Here's how the part is built. I have some questions about the finished solid (model axes, mm). Coordinates: 2 decimals unless noted, no trailing zeros. Write each loop counter-clockwise with the first axis right and the second up, starting at its lowest first coordinate (ties: lowest second). Pieces come first, ordered by that corner, then holes.
Item 1: Please list where these lines run through material, in increasing order: line 1 (Z direction, x = -30, y = 2.25); line 2 (Z direction, x = -8, y = 1.1); line 3 (X direction, y = 1.9, z = 8).
Item 2: I'm going to push a flat-ended pin straight in: P1, Ø5, axis at x = -62, z = 11, coming from the +Y side. Where does the tip first touch, or does it pass through?
Item 3: I want a section at A-A (x = -8). Please give me the cut outline in (y, z), and give its area (3 significant figures).
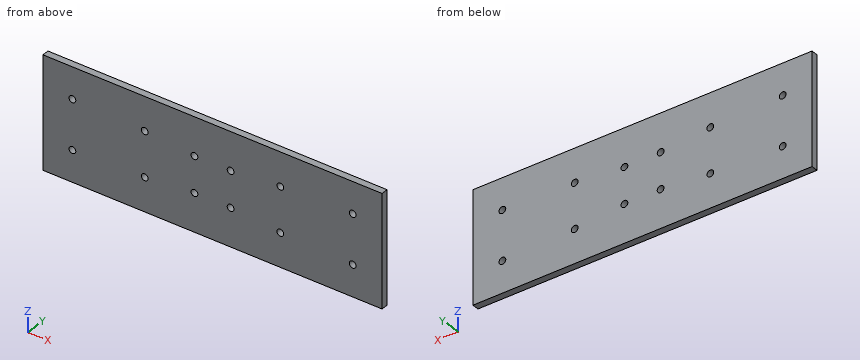
Autodesk Inventor part; units mm, degrees
ref_plane "YZ Plane" through (0, 0, 0) normal (1, 0, 0) x (0, 1, 0)
ref_plane "XZ Plane" through (0, 0, 0) normal (0, 1, 0) x (-1, 0, 0)
ref_plane "XY Plane" through (0, 0, 0) normal (0, 0, 1) x (1, 0, 0)
sketch "Szkic1" plane through (0, 0, 0) normal (0, 1, 0) x (-1, 0, 0)
  line L0 (75, 25) -> (-75, 25)
  line L1 (-75, 25) -> (-75, -25)
  line L2 (-75, -25) -> (75, -25)
  line L3 (75, -25) -> (75, 25)
  line L4 (75, 25) -> (-75, -25) construction
  line L5 (-75, 25) -> (75, -25) construction
  point P0 (0, 0)
  dimension "d0" = 150
  dimension "d1" = 50
extrude "Wyciągnięcie proste1" add sketch "Szkic1" along normal blind 3
sketch "Szkic3" plane through (0, 3, 0) normal (0, 1, 0) x (1, 0, 0)
  line L0 (75, 25) -> (-75, 25)
  line L1 (0, 25) -> (0, -25) construction
  line L2 (-75, -25) -> (75, -25)
  line L3 (-75, 25) -> (-75, -25)
  line L4 (-75, 0) -> (75, 0) construction
  line L5 (75, -25) -> (75, 25)
  point P0 (0, 0)
  point P1 (-30, 10)
  point P2 (30, 10)
  point P3 (-30, -10)
  point P4 (30, -10)
  dimension "d16" = 15
  dimension "d43" = 60
hole "Otwór2" at (-30, 3, -10) at (30, 3, -10) at (-30, 3, 10) at (30, 3, 10) direction (0, -1, 0) diameter 3 depth 8 tip angle 118
sketch "Szkic4" plane through (0, 3, 0) normal (0, 1, 0) x (1, 0, 0)
  line L0 (75, -25) -> (75, 25)
  line L1 (-75, 25) -> (-75, -25)
  line L2 (-75, 0) -> (75, 0) construction
  line L3 (75, 25) -> (-75, 25)
  line L4 (0, 25) -> (0, -25) construction
  point P0 (0, 0)
  point P1 (62, 11)
  point P2 (62, -11)
  point P3 (-62, 11)
  point P4 (-62, -11)
  dimension "d24" = 13
  dimension "d25" = 11
hole "Otwór3" at (62, 3, -11) at (62, 3, 11) at (-62, 3, -11) at (-62, 3, 11) direction (0, -1, 0) diameter 3 depth 8 tip angle 118
sketch "Szkic5" plane through (0, 3, 0) normal (0, 1, 0) x (1, 0, 0)
  line L0 (-8, -8) -> (8, -8)
  line L1 (8, -8) -> (8, 8)
  line L2 (8, 8) -> (-8, 8)
  line L3 (-8, 8) -> (-8, -8)
  line L4 (-8, -8) -> (8, 8) construction
  line L5 (8, -8) -> (-8, 8) construction
  point P0 (0, 0)
  dimension "d33" = 16
  dimension "d34" = 16
hole "Otwór4" at (-8, 3, -8) at (8, 3, -8) at (8, 3, 8) at (-8, 3, 8) direction (0, -1, 0) diameter 3 depth 8 tip angle 118
properties part number "Góra" material "Aluminium 6061"
Answer:
1. line 1: z = -25 to -11.5, -8.5 to 8.5, 11.5 to 25
1. line 2: z = -25 to -9.5, -6.5 to 6.5, 9.5 to 25
1. line 3: x = -75 to -9.5, -6.5 to 6.5, 9.5 to 75
2. P1: stops at y = 3
3. outline: (0, -25) - (3, -25) - (3, -9.5) - (0, -9.5) - close; (0, -6.5) - (3, -6.5) - (3, 6.5) - (0, 6.5) - close; (0, 9.5) - (3, 9.5) - (3, 25) - (0, 25) - close
3. area: 132 mm2
